Build history of the part. All positions in model axes, mm. A direction names the side the tool comes from. Give positions to 0.01 mm unless a question says otherwise; leave off trailing zeros. Write each loop counter-clockwise with the first axis right and the second up, starting at its lowest first coordinate (ties: lowest second). Pieces come first, ordered by that corner, then holes. Notation, with made-up numbers: (29, 54) -> (67, 54) arc R26 cw to (67, 73) -> close; hole circle Ø1 at (26, 30). An arc over 180 degrees is marked (long way). Write item = value, one per line. Start each with the question number.
Q1. Saw through at A-A, the plane y = 16.5. List the corners of the cut face in (x, z).
Q2. Tool access for faces 5 (the face through (83.802, 30.594, -23.069)), 6 (the face through (-57.905, 0.493, 0.867)): list every direction of +Z, -Z, +X, -X, +Y, -Y with a clear straight run to the whole face (end or side of a thin tool).
Q3. Mould opens along Z. For faces 1 (the face through (104, 30, -24)), 2 (the face through (61, 31, -85)), 3 (the face through (60, 30, -86)), 4 (the face through (104, 31, -25)) say: pulls with the +Z half, pulls with the -Z half, needs draft (parallel to the pull), parting line crosses it, or undercut.
Q4. Wall check: line 1 (X direction, y = 0.75, z = 0); line 2 (Z direction, x = 0, y = 23); line 3 (X direction, y = 0.7, z = 0). Give the ranges that are in metal, low to high.
Q5. Drop flat-ended pins along their axis: P1, Ø10, axis at x = -5.5, z = -49, coming from the -Y side; P2, Ø8, axis at y = 19, z = -62, coming from the -X side; P3, Ø8, axis at x = 26, z = 45.5, coming from the +Y side; P4, Ø12, axis at x = -26, y = 44, coming from the +Z side. Give the stop position or say it passes through.
from build123d import *

# Parameters (mm, degrees)
BOSS_EXTRUDE1_DEPTH = 1
BOSS_EXTRUDE2_DEPTH = 60
SKETCH2_R           = 6.5
CUT_EXTRUDE1_DEPTH  = 1
FILLET1_R           = 1
SKETCH3_R           = 4
CUT_EXTRUDE2_DEPTH  = 1


with BuildPart() as part:
    # Sketch1 → Boss-Extrude1 (new body)
    with BuildSketch(Plane(origin=(0, 0, 0), x_dir=(1, 0, 0), z_dir=(0, 1, 0))):
        with BuildLine():
            Line((121, 24), (121, 86))
            Line((121, 86), (0, 86))
            ThreePointArc((0, 86), (-53.630422544, -67.229292557), (83.849659702, 19.111111111))
            ThreePointArc((83.849659702, 19.111111111), (84.622700034, 22.494438258), (87.749643874, 24))
            Line((87.749643874, 24), (121, 24))
        make_face()
    extrude(amount=BOSS_EXTRUDE1_DEPTH)

    # Sketch1<3> → Boss-Extrude2 (add)
    with BuildSketch(Plane(origin=(0, 0, 0), x_dir=(1, 0, 0), z_dir=(0, 1, 0))):
        with BuildLine():
            ThreePointArc((87.749643874, 24), (84.622700034, 22.494438258), (83.849659702, 19.111111111))
            ThreePointArc((83.849659702, 19.111111111), (-53.630422544, -67.229292557), (0, 86))
            Line((0, 86), (121, 86))
            Line((121, 86), (121, 85))
            Line((121, 85), (120, 85))
            Line((120, 85), (0, 85))
            ThreePointArc((0, 85), (-53.006812979, -66.447556597), (82.874663659, 18.888888889))
            ThreePointArc((82.874663659, 18.888888889), (83.840964074, 23.118047822), (87.749643874, 25))
            Line((87.749643874, 25), (120, 25))
            Line((120, 25), (121, 25))
            Line((121, 25), (121, 24))
            Line((121, 24), (87.749643874, 24))
        make_face()
    extrude(amount=BOSS_EXTRUDE2_DEPTH)

    # Sketch2 → Cut-Extrude1 (cut)
    with BuildSketch(Plane(origin=(0, 1, 0), x_dir=(1, 0, 0), z_dir=(0, 1, 0))):
        with Locations(Location((0, 0, 0), (0, 0, 270))):
            Circle(SKETCH2_R)
    extrude(amount=-CUT_EXTRUDE1_DEPTH, mode=Mode.SUBTRACT)

    # Fillet1
    fillet1_edges = [part.edges().sort_by_distance(p)[0] for p in [
        (104.374821937, 1, -25),
        (83.840964074, 1, -23.118047822),
        (60.5, 1, -85),
        (60.5, 0, -86),
        (104.374821937, 0, -24),
        (84.622700034, 0, -22.494438258),
        (60.5, 60, -86),
        (104.374821937, 60, -24),
        (84.622700034, 60, -22.494438258),
        (-53.006812979, 1, 66.447556597),
        (-53.630422544, 0, 67.229292557),
        (-53.630422544, 60, 67.229292557),
    ]]
    fillet(fillet1_edges, radius=FILLET1_R - 0.0001)  # a hair under: the kernel refuses the full size

    # Sketch3 → Cut-Extrude2 (cut)
    with BuildSketch(Plane.XZ):
        with Locations(Location((-54, 0, 0), (0, 0, 270))):
            Circle(SKETCH3_R)
        with Locations(Location((54, 0, 0), (0, 0, 270))):
            Circle(SKETCH3_R)
    extrude(amount=-CUT_EXTRUDE2_DEPTH, mode=Mode.SUBTRACT)


solid = part.part
Report:
q1.outline = (0, -86) -> (121, -86) -> (121, -85) -> (0, -85) arc R85 cw (long way) to (82.87, -18.89) arc R5 ccw to (87.75, -25) -> (121, -25) -> (121, -24) -> (87.75, -24) arc R4 cw to (83.85, -19.11) arc R86 ccw (long way) to start
q2.face_5 = +Y
q2.face_6 = +Y, -Y
q3.face_1 = pulls with the +Z half
q3.face_2 = undercut
q3.face_3 = pulls with the -Z half
q3.face_4 = undercut
q4.line_1 = -85.97 to -58, -50 to -6.5, 6.5 to 50, 58 to 85.97
q4.line_2 = -86 to -85, 85 to 86
q4.line_3 = -85.95 to -58, -50 to -6.5, 6.5 to 50, 58 to 85.95
q5.P1 = 0
q5.P2 = -63.5
q5.P3 = 1
q5.P4 = 83.64
